Design review of the part built by this model. Coordinates are the model's own, in mm. Face numbers are marked on the shaded views. A direction names the side the tool comes from. Round coordinates to 2 decimals unless told otherwise and drop trailing zeros. Order: outer loops, then holes, each group sorted by start corner. A loop starts at its lowest first (then second) coordinate and runs counter-clockwise, first axis right, second up. Notation, with made-up numbers: (-16.75, -21) - (-11.75, -21) arc R35 ccw to (-11.75, 18) - close; hole circle Ø9 at (-14.75, 24). An arc over 180 degrees is marked (long way). Use CSV: the item, a comma, the result in double quotes.
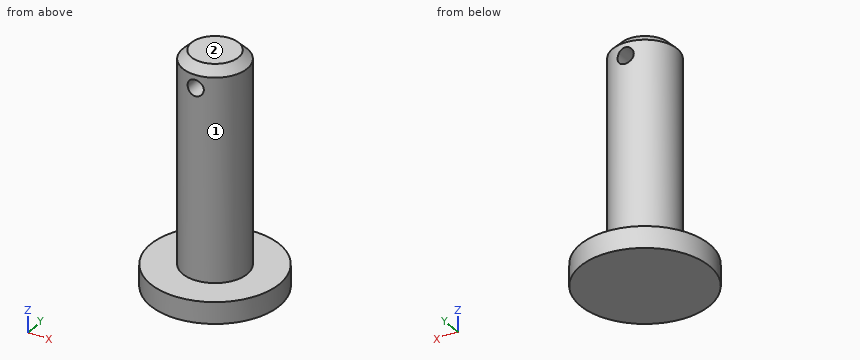
from build123d import *

# Parameters (mm, degrees)
F0_R     = 19.05
F1_DEPTH = 6.35
F2_R     = 9.525
F3_DEPTH = 62.23
F4_SIZE  = 2.54
F5_R     = 2.3876
F6_DEPTH = 12.7


with BuildPart() as f1:
    # F0 (on Top) → F1 (new body)
    with BuildSketch(Plane.XY):
        Circle(F0_R)
    extrude(amount=F1_DEPTH)

    # F2 (on face) → F3 (join)
    with BuildSketch(Plane.XY.offset(6.35)):
        Circle(F2_R)
    extrude(amount=F3_DEPTH)

    # F4
    f4_edges = [f1.edges().sort_by_distance(p)[0] for p in [
        (-9.525, 0, 68.58),
    ]]
    chamfer(f4_edges, length=F4_SIZE)

    # F5 (on Front) → F6 (cut, symmetric)
    with BuildSketch(Plane.XZ):
        with Locations((0, 62.23)):
            Circle(F5_R)
    extrude(amount=F6_DEPTH, both=True, mode=Mode.SUBTRACT)


solid = f1.part
1) For the marked faces 1 and 2, list the 3-axis set-ups (+Z, -Z, +X, -X, +Y, -Y) from which the entire face can be reached by the end or side of a thin tool; tool diameter is ignored.
Data:
face 1,"+Z"
face 2,"+Z, +X, -X, +Y, -Y"
2) We need section A-A (y = 0). Give the boundary of the cut face in (x, z) (3 decimals), then the cut area to 3 significant figures.
Data:
outline,"(-19.05, 0) - (19.05, 0) - (19.05, 6.35) - (9.525, 6.35) - (9.525, 66.04) - (6.985, 68.58) - (-6.985, 68.58) - (-9.525, 66.04) - (-9.525, 6.35) - (-19.05, 6.35) - close; hole circle Ø4.775 at (0, 62.23)"
area,"1,400 mm2"
3) We need section C-C (x = -14). Give the boundary of the cut face in (y, z), then the cut area to 3 significant figures.
Data:
outline,"(-12.92, 0) - (12.92, 0) - (12.92, 6.35) - (-12.92, 6.35) - close"
area,"164 mm2"
4) We need section B-B (z = 63). Give the boundary of the cut face in (x, y) (3 decimals), then the cut area to 3 significant figures.
Data:
outline,"(-2.26, -9.253) - (-2.26, 9.253) arc R9.525 ccw to start; (2.26, -9.253) arc R9.525 ccw to (2.26, 9.253) - close"
area,"200 mm2"
5) Insertion check: pin 1 Ø1.5 at (x, z) = (-2.5, 28) entering from +Y; pin 2 Ø1.5 at (y, z) = (-4, 16) entering from +X; pin 3 Ø8 at (y, z) = (-3.5, 25.5) entering from -X (3 decimals); pin 4 Ø4 at (x, y) = (1.5, 11) entering from -Z. Each pin has a flat end and moves straight along its axis. Give the tip position at first contact, or say it passes through.
Data:
pin 1,"stops at y = 9.36"
pin 2,"stops at x = 8.95"
pin 3,"stops at x = -9.525"
pin 4,"stops at z = 0"
6) We need section D-D (y = -12). Give the boundary of the cut face in (x, z).
Data:
outline,"(-14.8, 0) - (14.8, 0) - (14.8, 6.35) - (-14.8, 6.35) - close"
7) To check wall thickness, follow L1, parallel to Z at x = 0, y = -1.25; L2, parallel to Z at x = 2, y = 10.5; L3, parallel to X at y = -4.25, z = 62.23. State the ranges of each line that lie inside material, in increasing order. Write a range as from..to.
Data:
L1,"z = 0..59.84, 64.62..68.58"
L2,"z = 0..6.35"
L3,"x = -8.52..-2.39, 2.39..8.52"
